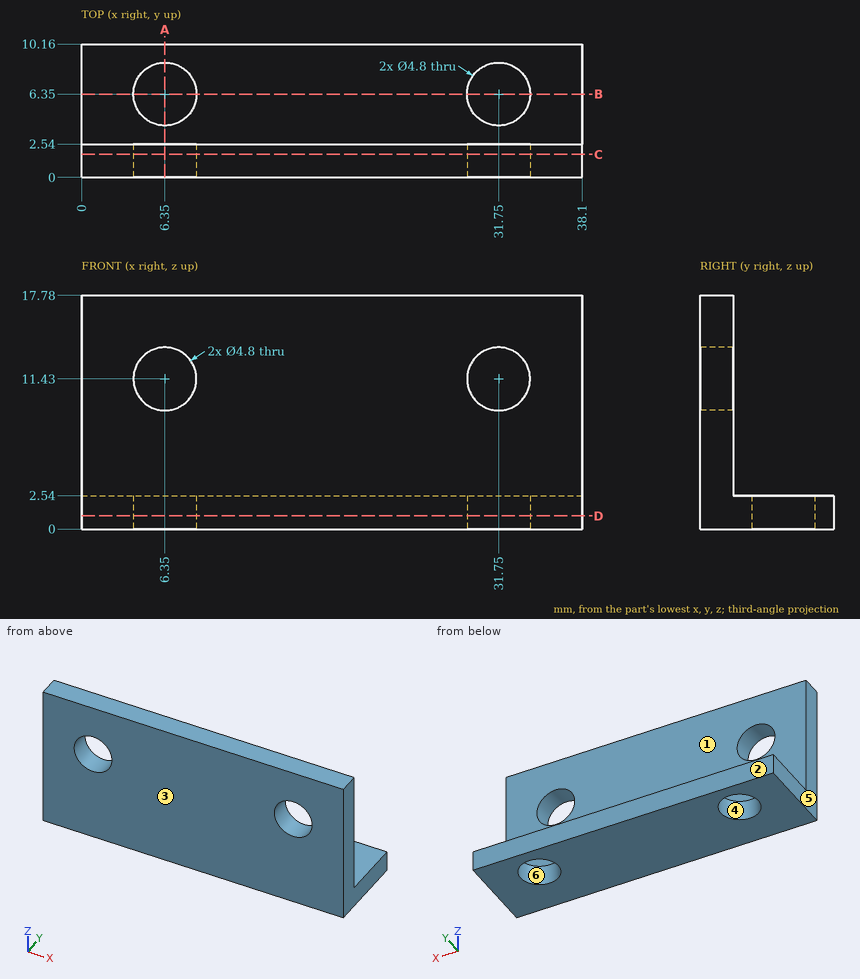
Print and shaded views of the part. All mm, measured from the part's lowest x, y and z. A direction names the side the tool comes from. Give positions to 0.01 mm unless a question says otherwise; leave off trailing zeros. Loops run counter-clockwise (first coordinate to the right, second up) from the corner with the lowest first, then second, coordinate; pieces in that order, holes last. Notation, with made-up numbers: (6.25, 61.25) -> (18.25, 61.25) arc R16 ccw to (18.25, 87.25) -> close; hole circle Ø10 at (0.5, -8.5). An arc over 180 degrees is marked (long way). Answer in a Markdown table with one row per item.
Item 1: Flat gauge pins, fed straight in: P1, Ø4, axis at x = 25.5, y = 5, coming from the +Z side; P2, Ø5, axis at x = 12.5, z = 7, coming from the +Y side; P3, Ø5, axis at x = 19, z = 11.5, coming from the -Y side. Where does each tip first touch, or does it go through?
Findings below:
| item | result |
|---|---|
| P1 | stops at z = 2.54 |
| P2 | stops at y = 2.54 |
| P3 | stops at y = 0 |
Item 2: Slice it at D-D on z = 1. Write the cut outline in (x, y), plus the area to 3 significant figures.
Findings below:
| item | result |
|---|---|
| outline | (0, 0) -> (38.1, 0) -> (38.1, 10.16) -> (0, 10.16) -> close; hole circle Ø4.8 at (6.35, 6.35); hole circle Ø4.8 at (31.75, 6.35) |
| area | 351 mm² |
Item 3: Mould opens along X. For the marked faces 3, 4, 5 and 6 say: pulls with the +X half, pulls with the -X half, needs draft (parallel to the pull), parting line crosses it, or undercut.
Findings below:
| item | result |
|---|---|
| face 3 | needs draft |
| face 4 | undercut |
| face 5 | pulls with the -X half |
| face 6 | undercut |
Item 4: Probe line 1 along Y through (x, z) = (6.35, 1.45); line 2 along X through (y, z) = (1.75, 13.5); line 3 along Z through (x, y) = (31.75, 0.7). List the from-to ranges inside material, lowest first. Write a range as [from, to].
Findings below:
| item | result |
|---|---|
| line 1 | y = [0, 3.95], [8.75, 10.16] |
| line 2 | x = [0, 5.14], [7.56, 30.54], [32.96, 38.1] |
| line 3 | z = [0, 9.03], [13.83, 17.78] |
Item 5: Slice it at B-B on y = 6.35. Write the cut outline in (x, z).
Findings below:
| item | result |
|---|---|
| outline | (0, 0) -> (3.95, 0) -> (3.95, 2.54) -> (0, 2.54) -> close; (8.75, 0) -> (29.35, 0) -> (29.35, 2.54) -> (8.75, 2.54) -> close; (34.15, 0) -> (38.1, 0) -> (38.1, 2.54) -> (34.15, 2.54) -> close |
Item 6: Tool access for the marked faces 1 and 2: list every direction of +Z, -Z, +X, -X, +Y, -Y with a clear straight run to the whole face (end or side of a thin tool).
Findings below:
| item | result |
|---|---|
| face 1 | +Z, +X, -X, +Y |
| face 2 | +Z, -Z, +X, -X, +Y |
Item 7: Slice it at A-A on x = 6.35. Write the cut outline in (y, z), plus the area to 3 significant figures.
Findings below:
| item | result |
|---|---|
| outline | (0, 0) -> (3.95, 0) -> (3.95, 2.54) -> (2.54, 2.54) -> (2.54, 9.03) -> (0, 9.03) -> close; (0, 13.83) -> (2.54, 13.83) -> (2.54, 17.78) -> (0, 17.78) -> close; (8.75, 0) -> (10.16, 0) -> (10.16, 2.54) -> (8.75, 2.54) -> close |
| area | 40.1 mm² |
Item 8: Slice it at C-C on y = 1.75. Write the cut outline in (x, z), plus the area to 3 significant figures.
Findings below:
| item | result |
|---|---|
| outline | (0, 0) -> (38.1, 0) -> (38.1, 17.78) -> (0, 17.78) -> close; hole circle Ø4.8 at (6.35, 11.43); hole circle Ø4.8 at (31.75, 11.43) |
| area | 641 mm² |
